Check sheet for the drawn part. Datum: minimum x, y, z corner. Units: mm. A direction names the side the tool comes from. Coordinates: 2 decimals unless noted, no trailing zeros. Order: outer loops, then holes, each group sorted by start corner. A loop starts at its lowest first (then second) coordinate and runs counter-clockwise, first axis right, second up. Notation, with made-up numbers: M 0.25,-20 L 58.25,-20 A22 ccw 58.25,-14 Z; hole C 16,-39 d2. An arc over 180 degrees is marked long. Use one line per item in the form item = value. Start each with the question number.
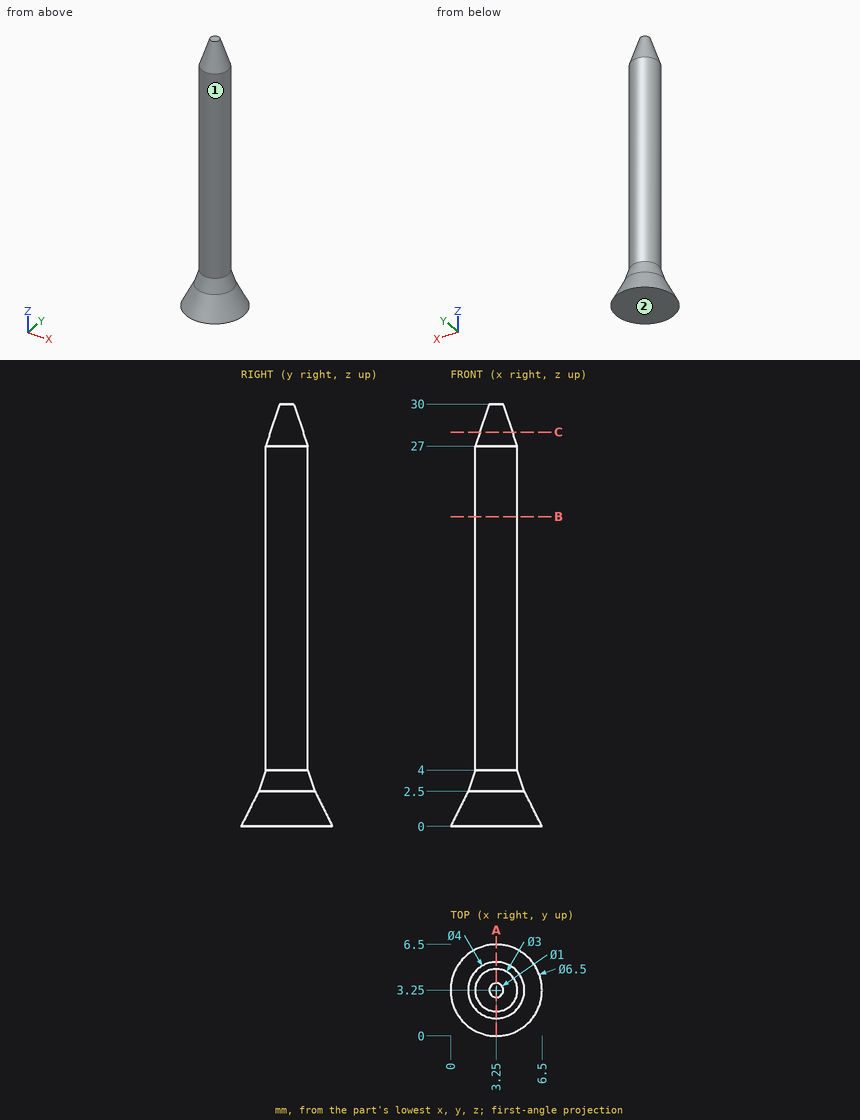
1. Cross-section at A-A on x = 3.25. Enter the section's corners in (y, z).
2. Tool access check on the marked faces 1 and 2. Record the directions out of +Z, -Z, +X, -X, +Y, -Y that give a thin tool (end or side, any length) a straight path to the whole face; none if there is none.
3. Cross-section at C-C on z = 28. Enter the section's corners in (x, y).
4. Material ranges on line 1 along X through (y, z) = (2.5, 1); line 2 along Z through (x, y) = (1.5, 5); line 3 along X through (y, z) = (2.5, 14), recorded low to high.
5. Cross-section at B-B on z = 22. Enter the section's corners in (x, y).
Final values:
q1.outline = M 0,0 L 6.5,0 L 5.25,2.5 L 4.75,4 L 4.75,27 L 3.75,30 L 2.75,30 L 1.75,27 L 1.75,4 L 1.25,2.5 Z
q2.face_1 = +Z
q2.face_2 = -Z, +X, -X, +Y, -Y
q3.outline = C 3.25,3.25 d2.33
q4.line_1 = 0.6 to 5.9
q4.line_2 = 0 to 1.55
q4.line_3 = 1.95 to 4.55
q5.outline = C 3.25,3.25 d3
